Could you check a few things on this model? Use its own coordinates, in mm. Face numbers are marked on the shaded views. A direction names the side the tool comes from. Coordinates: 2 decimals unless noted, no trailing zeros. Loops run counter-clockwise (first coordinate to the right, second up) from the corner with the lowest first, then second, coordinate; pieces in that order, holes last. Notation, with made-up numbers: (75, 70.25) -> (133, 70.25) arc R4 cw to (133, 74.25) -> close; hole circle Ø4 at (84, 23). An arc over 180 degrees is marked (long way). One line per question, with ' | ' between items.
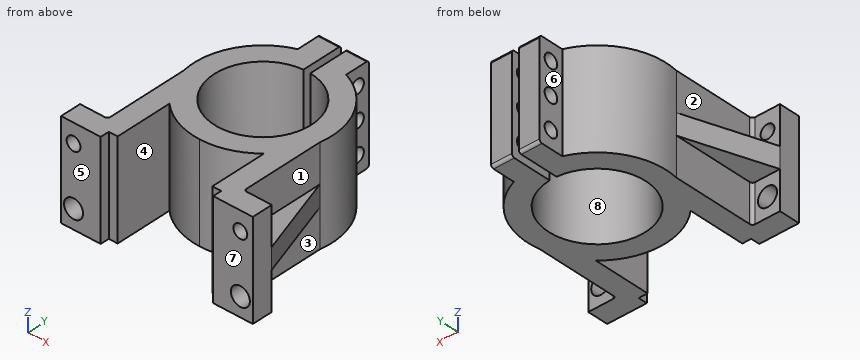
```python
from build123d import *
from build123d.topology import SkipClean

# Parameters (mm, degrees)
BOSS_EXTRUDE1_DEPTH  = 28
BOSS_EXTRUDE2_START  = 11
BOSS_EXTRUDE2_DEPTH  = 6
CUT_EXTRUDE1_REACH   = 50.35
SKETCH3_R            = 2
FILLET1_R            = 0.8
SKETCH4_R            = 2
SKETCH4_R_2          = 2.75
CUT_EXTRUDE2_DEPTH   = 67.419950062
FILLET1_OF_MIRROR1_R = 0.8
CUT_EXTRUDE3_DEPTH   = 52.732976543


with BuildPart() as part:
    # Sketch1 → Boss-Extrude1 (new body)
    with BuildSketch(Plane.XY):
        with BuildLine():
            Line((0, 20), (0, 14))
            ThreePointArc((0, 14), (14, 0), (0, -14))
            Line((0, -14), (0, -20))
            ThreePointArc((0, -20), (7.356284672, -18.5979858), (13.681207787, -14.588507583))
            Line((13.681207787, -14.588507583), (13.681207787, -30.99669229))
            Line((13.681207787, -30.99669229), (16.241207787, -30.99669229))
            Line((16.241207787, -30.99669229), (16.241207787, -33.55669229))
            Line((16.241207787, -33.55669229), (27.681207787, -33.55669229))
            Line((27.681207787, -33.55669229), (27.681207787, -27.55669229))
            Line((27.681207787, -27.55669229), (20.481207787, -27.55669229))
            ThreePointArc((20.481207787, -27.55669229), (19.915522362, -27.322377715), (19.681207787, -26.75669229))
            Line((19.681207787, -26.75669229), (19.681207787, -3.55669229))
            ThreePointArc((19.681207787, -3.55669229), (17.38394465, 9.889310815), (7, 18.734993995))
            Line((7, 18.734993995), (7, 25.934993995))
            Line((7, 25.934993995), (0, 25.934993995))
            Line((0, 25.934993995), (0, 20))
        make_face()
    boss_extrude1 = extrude(amount=BOSS_EXTRUDE1_DEPTH)

    # Sketch2 → Boss-Extrude2 (add)
    with BuildSketch(Plane.XY.offset(BOSS_EXTRUDE2_START)):
        Polygon((19.681207787, -26.75669229), (19.681207787, -3.55669229), (27.681207787, -27.55669229), (20.481207787, -27.55669229), (19.681207787, -27.55669229), align=None)
    boss_extrude2 = extrude(amount=BOSS_EXTRUDE2_DEPTH)

    # Sketch3 → Cut-Extrude1 (cut, up to next)
    with BuildSketch(Plane(origin=(7, 0, 0), x_dir=(0, 0, -1), z_dir=(1, 0, 0)), mode=Mode.PRIVATE) as cut_extrude1_sk1:
        with Locations(Location((-23, 22.334993995, 0), (0, 0, 90))):
            Circle(SKETCH3_R)
    cut_extrude1_tool1 = extrude(cut_extrude1_sk1.sketch, amount=-CUT_EXTRUDE1_REACH, mode=Mode.PRIVATE) & part.part
    # Sketch3 → Cut-Extrude1 (cut, up to next)
    with BuildSketch(Plane(origin=(7, 0, 0), x_dir=(0, 0, -1), z_dir=(1, 0, 0)), mode=Mode.PRIVATE) as cut_extrude1_sk2:
        with Locations(Location((-14, 22.334993995, 0), (0, 0, 90))):
            Circle(SKETCH3_R)
    cut_extrude1_tool2 = extrude(cut_extrude1_sk2.sketch, amount=-CUT_EXTRUDE1_REACH, mode=Mode.PRIVATE) & part.part
    # Sketch3 → Cut-Extrude1 (cut, up to next)
    with BuildSketch(Plane(origin=(7, 0, 0), x_dir=(0, 0, -1), z_dir=(1, 0, 0)), mode=Mode.PRIVATE) as cut_extrude1_sk3:
        with Locations(Location((-5, 22.334993995, 0), (0, 0, 90))):
            Circle(SKETCH3_R)
    cut_extrude1_tool3 = extrude(cut_extrude1_sk3.sketch, amount=-CUT_EXTRUDE1_REACH, mode=Mode.PRIVATE) & part.part
    cut_extrude1_1 = cut_extrude1_tool1.solids().sort_by_distance((7, 22.334994, 23))[0]
    add(cut_extrude1_1, mode=Mode.SUBTRACT)
    cut_extrude1_2 = cut_extrude1_tool2.solids().sort_by_distance((7, 22.334994, 14))[0]
    add(cut_extrude1_2, mode=Mode.SUBTRACT)
    cut_extrude1_3 = cut_extrude1_tool3.solids().sort_by_distance((7, 22.334994, 5))[0]
    add(cut_extrude1_3, mode=Mode.SUBTRACT)
    cut_extrude1 = cut_extrude1_1 + cut_extrude1_2 + cut_extrude1_3  # Cut-Extrude1 as one shape, for the pattern or mirror that repeats it

    # Fillet1
    fillet1_edges = [part.edges().sort_by_distance(p)[0] for p in [
        (3.5, 25.934993995, 0),
        (3.5, 25.934993995, 28),
    ]]
    fillet(fillet1_edges, radius=FILLET1_R)

    # Sketch4 → Cut-Extrude2 (cut, through all)
    with BuildSketch(Plane(origin=(0, -27.55669229, 0), x_dir=(1, 0, 0), z_dir=(0, 1, 0))):
        with Locations(Location((24.081207787, -22.5, 0), (0, 0, 270))):
            Circle(SKETCH4_R)
        with Locations(Location((24.081207787, -5.5, 0), (0, 0, 270))):
            Circle(SKETCH4_R_2)
    cut_extrude2 = extrude(amount=-CUT_EXTRUDE2_DEPTH, mode=Mode.SUBTRACT)

    # Mirror1: Boss-Extrude1, Boss-Extrude2, Cut-Extrude1, Cut-Extrude2 across plane
    with SkipClean():  # the faces are left unmerged after this step: merging them gives an invalid solid
        add(boss_extrude1.mirror(Plane(origin=(0, 0, 0), x_dir=(0, 0, 1), z_dir=(1, 0, 0))))
        add(boss_extrude2.mirror(Plane(origin=(0, 0, 0), x_dir=(0, 0, 1), z_dir=(1, 0, 0))))
        add(cut_extrude1.mirror(Plane(origin=(0, 0, 0), x_dir=(0, 0, 1), z_dir=(1, 0, 0))), mode=Mode.SUBTRACT)
        add(cut_extrude2.mirror(Plane(origin=(0, 0, 0), x_dir=(0, 0, 1), z_dir=(1, 0, 0))), mode=Mode.SUBTRACT)

    # Fillet1 of Mirror1
    fillet1_of_mirror1_edges = [part.edges().sort_by_distance(p)[0] for p in [
        (-3.5, 25.934993995, 0),
        (-3.5, 25.934993995, 28),
    ]]
    fillet(fillet1_of_mirror1_edges, radius=FILLET1_OF_MIRROR1_R)

    # Sketch6 → Cut-Extrude3 (cut, through all)
    with BuildSketch(Plane.XY.offset(28)):
        with BuildLine():
            ThreePointArc((1, 13.964240044), (0, 14), (-1, 13.964240044))
            Line((-1, 13.964240044), (-1, 8.456424639))
            Line((-1, 8.456424639), (1, 8.456424639))
            Line((1, 8.456424639), (1, 13.964240044))
        make_face()
        with BuildLine():
            Line((-1, 8.456424639), (-1, 13.964240044))
            ThreePointArc((-1, 13.964240044), (-9.539392014, -10.246950766), (14, 0))
            ThreePointArc((14, 0), (10.246950766, 9.539392014), (1, 13.964240044))
            Line((1, 13.964240044), (1, 8.456424639))
            Line((1, 8.456424639), (-1, 8.456424639))
        make_face()
        with BuildLine():
            Line((0, 25.134993995), (-1, 25.134993995))
            Line((-1, 25.134993995), (-1, 13.964240044))
            ThreePointArc((-1, 13.964240044), (0, 14), (1, 13.964240044))
            Line((1, 13.964240044), (1, 25.134993995))
            Line((1, 25.134993995), (0, 25.134993995))
        make_face()
        Polygon((1, 41.813563352), (-1, 41.813563352), (-1, 25.134993995), (0, 25.134993995), (1, 25.134993995), align=None)
    extrude(amount=-CUT_EXTRUDE3_DEPTH, mode=Mode.SUBTRACT)


solid = part.part
```
Q1. For pin 1 (2.5 mm diameter, centred on x = 22.5, y = -10.5, fed in from +Z); pin 2 (1.5 mm diameter, centred on y = -6.5, z = 11, fed in from +X); pin 3 (6 mm diameter, centred on y = 20, z = 3.5, fed in from -X), each with a flat end and sliding along its axis, tell me the tip position at first contact or that it passes through.
Values follow:
pin 1: stops at z = 17 | pin 2: stops at x = 20.91 | pin 3: stops at x = -10.54
Q2. We'd pull the mould along Y, two halves only. Please class the marked faces 6, 7 and 8: released by +Y, released by -Y, zero draft, split by the parting line, or undercut.
Values follow:
face 6: zero draft | face 7: released by -Y | face 8: undercut
Q3. Imagine slicing it at C-C on y = 15. Write out the boundary of the cut face in (x, z), plus the area to 3 significant figures.
Values follow:
outline: (-13.23, 0) -> (-1, 0) -> (-1, 28) -> (-13.23, 28) -> close; (1, 0) -> (13.23, 0) -> (13.23, 28) -> (1, 28) -> close | area: 685 mm2
Q4. Imagine slicing it at B-B on x = -12. Write out the boundary of the cut face in (y, z).
Values follow:
outline: (-16, 0) -> (-7.21, 0) -> (-7.21, 28) -> (-16, 28) -> close; (7.21, 0) -> (16, 0) -> (16, 28) -> (7.21, 28) -> close
Q5. Imagine slicing it at A-A on z = 14. Give the number of separate pieces and of enclosed holes in the cut face, plus the area to 3 significant figures.
Values follow:
separate pieces: 3 | enclosed holes: 0 | area: 1,210 mm2
Q6. For the marked faces 1, 2, 3, 4 and 5, which set-ups out of +Z, -Z, +X, -X, +Y, -Y let a thin tool reach every point of the face, with its end or its side?
Values follow:
face 1: +Z, +X | face 2: +Z, -X | face 3: -Z, +X | face 4: +Z, -Z, -Y | face 5: +Z, -Z, +X, -X, -Y
Q7. Imagine slicing it at D-D on z = 10. Write out the boundary of the cut face in (x, y) (1 decimal).
Values follow:
outline: (-27.7, -33.6) -> (-16.2, -33.6) -> (-16.2, -31) -> (-13.7, -31) -> (-13.7, -14.6) arc R20 ccw to (13.7, -14.6) -> (13.7, -31) -> (16.2, -31) -> (16.2, -33.6) -> (27.7, -33.6) -> (27.7, -27.6) -> (20.5, -27.6) arc R0.8 cw to (19.7, -26.8) -> (19.7, -3.6) arc R20 ccw to (7, 18.7) -> (7, 25.9) -> (1, 25.9) -> (1, 14) arc R14 cw (long way) to (-1, 14) -> (-1, 25.9) -> (-7, 25.9) -> (-7, 18.7) arc R20 ccw to (-19.7, -3.6) -> (-19.7, -26.8) arc R0.8 cw to (-20.5, -27.6) -> (-27.7, -27.6) -> close
Q8. Please list where these lines run through material, in increasing order: L1, parallel to X at y = -25, z = 7; L2, parallel to X at y = -28.95, z = 22.5; L3, parallel to Y at x = -4.4, z = 5 (3 decimals). Write a range as [from, to].
Values follow:
L1: x = [-19.68, -13.68], [13.68, 19.68] | L2: x = [-27.68, -26.08], [-22.08, -13.68], [13.68, 22.08], [26.08, 27.68] | L3: y = [-19.51, -13.291], [13.291, 20.335], [24.335, 25.935]
